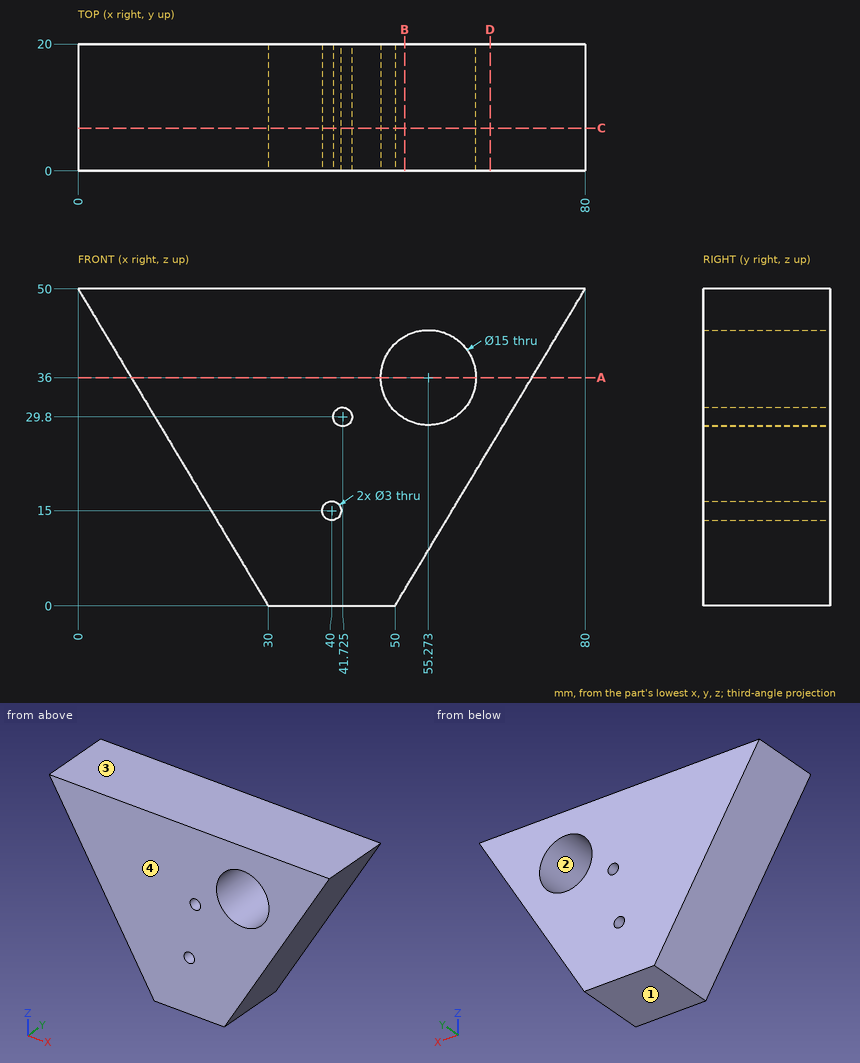
Geometry: see drawing. Coordinates: mm, zero at the bounding-box minimum. Coordinates: 2 decimals unless noted, no trailing zeros. Order: outer loops, then holes, each group sorted by start corner. A loop starts at its lowest first (then second) coordinate and runs counter-clockwise, first axis right, second up. Notation, with made-up numbers: (15.5, 63.25) - (21.5, 63.25) arc R29 ccw to (21.5, 88.25) - close; hole circle Ø1 at (-1.75, -10). An arc over 180 degrees is marked (long way). Write each question's results on one line, items separated by ' | '.
(1) Section query B-B, the plane x = 51.5. Return the cut outline in (y, z).
Values found:
outline: (0, 2.5) - (20, 2.5) - (20, 29.52) - (0, 29.52) - close; (0, 42.48) - (20, 42.48) - (20, 50) - (0, 50) - close
(2) Section query A-A, the plane z = 36. Return the cut outline in (x, y), plus the area to 3 significant figures.
Values found:
outline: (8.4, 0) - (47.77, 0) - (47.77, 20) - (8.4, 20) - close; (62.77, 0) - (71.6, 0) - (71.6, 20) - (62.77, 20) - close | area: 964 mm²
(3) First-contact query: pin 1 Ø12 at (x, y) = (9, 17) entering from -Z; pin 2 Ø5 at (x, z) = (52, 7.5) entering from -Y; pin 3 Ø5 at (y, z) = (6.5, 24.5) entering from -X; pin 4 Ø2 at (x, y) = (71, 13.5) entering from -Z (1 decimal). Flat tips, straight axial feed; report the tip coordinate or a pass-through.
Values found:
pin 1: stops at z = 25 | pin 2: stops at y = 0 | pin 3: stops at x = 13.8 | pin 4: stops at z = 33.3
(4) Line query: line 1 (Z direction, x = 40, y = 4.75); line 2 (X direction, y = 5.75, z = 32.5) (1 decimal); line 3 (Z direction, x = 39.5, y = 8.25) (1 decimal). Output: solid intervals per line, ascending. Write a range as [from, to].
Values found:
line 1: z = [0, 13.5], [16.5, 50] | line 2: x = [10.5, 48.6], [61.9, 69.5] | line 3: z = [0, 13.6], [16.4, 50]
(5) Section query D-D, the plane x = 65. Return the cut outline in (y, z).
Values found:
outline: (0, 25) - (20, 25) - (20, 50) - (0, 50) - close
(6) Mould query, pull axis Z, two halves, no side actions, for the marked faces 1, 2, 3 and 4. Classes: +Z half, -Z half, draft (parallel to the pull), parting line (faces both ways), or undercut.
Values found:
face 1: -Z half | face 2: undercut | face 3: +Z half | face 4: draft
(7) Section query C-C, the plane y = 6.75. Return the cut outline in (x, z) (1 decimal), plus the area to 3 significant figures.
Values found:
outline: (0, 50) - (30, 0) - (50, 0) - (80, 50) - close; hole circle Ø3 at (40, 15); hole circle Ø3 at (41.7, 29.8); hole circle Ø15 at (55.3, 36) | area: 2,310 mm²
